Source: CAD feature listing. Evaluate the final solid. Frame: model axes, mm. A direction names the side the tool comes from. Coordinates: 2 decimals unless noted, no trailing zeros. Order: outer loops, then holes, each group sorted by start corner. A loop starts at its lowest first (then second) coordinate and runs counter-clockwise, first axis right, second up. Notation, with made-up numbers: (-14.75, 84.25) - (-7.75, 84.25) arc R8 cw to (-7.75, 99.25) - close; hole circle Ø6 at (-25.75, -10). An arc over 180 degrees is marked (long way). One line per question, with ' | ' between items. Start each with the question number.
(1) Draft query along X for faces 3 (the flat face through (-3.523, -2.068, 0.986)), 4 (the flat face through (0, -3, 0)), 5 (the cylindrical face through (-0.342, 1.442, 0.986)), 6 (the cylindrical face through (-0.09, 2.99, 0.99)). Return one class per face: +X half, -X half, draft (parallel to the pull), parting line (faces both ways), or undercut.
(2) Line query: line 1 along Z through (x, y) = (1.5, -8.75); line 2 along Y through (x, z) = (1, 0.85); line 3 along Y through (x, z) = (-1.25, 1.8). Output: solid intervals per line, ascending.
(3) Section B-B (y = -3). Return the cut outline in (x, z).
(4) Section C-C (y = 2). Return the cut outline in (x, z).
(5) Section A-A (z = 0.95). Return the cut outline in (x, y), then the cut area to 3 significant figures.
(6) Contact query for flat-ended pins moving along their axis: P1, Ø3, axis at x = 2.5, y = -1, coming from the +Z side; P2, Ø1.5, axis at x = 2.5, y = -4, coming from the +Z side. Output: stop coordinate, or through.
(7) Access query for faces 1 (the flat face through (3.5, -2.04, 0.99)), 2 (the flat face through (0, -2, 2)). Directions: +Z, -Z, +X, -X, +Y, -Y. A direction counts if a zero-diameter tool reaches every point of the face in a straight line with its end or side. Return the directions, or none.
Autodesk Inventor part; units mm, degrees
ref_plane "YZ Plane" through (0, 0, 0) normal (1, 0, 0) x (0, 1, 0)
ref_plane "XZ Plane" through (0, 0, 0) normal (0, 1, 0) x (-1, 0, 0)
ref_plane "XY Plane" through (0, 0, 0) normal (0, 0, 1) x (1, 0, 0)
sketch "Sketch1" plane through (0, 0, 0) normal (0, 0, 1) x (1, 0, 0)
  circle A0 centre (-0.0198, -0.0084) radius 1.4858
  arc A1 (0.0044, -3.1481) -> (0.0044, -8.2481) centre (0.0044, -5.6981) ccw construction
  arc A2 (0.0044, -8.2481) -> (0.0044, -3.1481) centre (0.0044, -5.6981) ccw construction
  line L0 (-5.8056, -3.1481) -> (0.0044, -3.1481) construction
  line L1 (0.0044, -8.2481) -> (-5.8056, -8.2481) construction
  line L2 (2.5544, -5.6981) -> (5.0544, -5.6981) construction
  line L3 (-5.8056, -3.1481) -> (-5.8056, -8.2481) construction
  arc A3 (2.9095, 0.6389) -> (-2.9546, 0.6139) centre (-0.0198, -0.0084) ccw
  arc A4 (-4.1081, -4.8261) -> (4.1094, -4.7911) centre (0.0044, -5.6981) ccw
  line L4 (2.9095, 0.6389) -> (4.1094, -4.7911)
  line L5 (-2.9546, 0.6139) -> (-4.1081, -4.8261)
  point P0 (0, 0)
  dimension "d0" = 2.5
  dimension "d1" = 6
extrude "Extrusion1" add sketch "Sketch1" along normal blind 2
sketch "Sketch2" plane through (0, 0, 2) normal (0, 0, 1) x (1, 0, 0)
  circle A0 centre (-0.0198, -0.0084) radius 1.4858
  arc A1 (0.0044, -3.1481) -> (0.0044, -8.2481) centre (0.0044, -5.6981) ccw construction
  arc A2 (0.0044, -8.2481) -> (0.0044, -3.1481) centre (0.0044, -5.6981) ccw construction
  line L0 (-5.8056, -3.1481) -> (0.0044, -3.1481) construction
  line L1 (0.0044, -8.2481) -> (-5.8056, -8.2481) construction
  line L2 (2.5544, -5.6981) -> (5.0544, -5.6981) construction
  line L3 (-5.8056, -3.1481) -> (-5.8056, -8.2481) construction
  arc A3 (2.9095, 0.6389) -> (-2.9546, 0.6139) centre (-0.0198, -0.0084) ccw
  arc A4 (-4.1081, -4.8261) -> (4.1094, -4.7911) centre (0.0044, -5.6981) ccw
  line L4 (2.9095, 0.6389) -> (4.1094, -4.7911)
  line L5 (-2.9546, 0.6139) -> (-4.1081, -4.8261)
  circle A5 centre (0.0044, -5.6981) radius 2.55
  point P0 (0, 0)
  point P1 (0, 0)
  dimension "d4" = 2.5
  dimension "d5" = 6
extrude "Extrusion2" add sketch "Sketch2" along normal blind 1.5 contours A5
fillet "Fillet1" radius 2.5 1 edges at (-2.5456, -5.6981, 3.5)
sketch "Sketch3" plane through (2.9095, 0.6389, 2) normal (0.9764456, 0.2157637, 0) x (0, 0, -1)
  line L0 (0, 3) -> (0, 0)
  line L1 (0, 0) -> (-1, 0)
  line L2 (-1, 0) -> (-1, -8.6875)
  line L3 (-1, -8.6875) -> (-2.9665, -8.6875)
  line L4 (-2.9665, -8.6875) -> (-2.9665, 0)
  line L5 (-2.9665, 0) -> (-1, 0)
  point P0 (2, 0.0039)
  point P1 (0, 1.2408)
  dimension "d9" = 1
extrude "Extrusion3" cut sketch "Sketch3" against normal blind 10
properties part number "Stylis holder"
Response values:
1) face 3: -X half | face 4: draft | face 5: undercut | face 6: parting line
2) line 1: z = 0 to 2 | line 2: y = -9.78 to -1.09, 1.07 to 2.81 | line 3: y = -9.71 to -0.84, 0.82 to 2.73
3) outline: (-3.72, 0) - (3.71, 0) - (3.71, 2) - (-3.72, 2) - close
4) outline: (-2.25, 0) - (2.21, 0) - (2.21, 2) - (-2.25, 2) - close
5) outline: (-4.11, -4.83) arc R4.2 ccw (long way) to (4.11, -4.79) - (2.91, 0.64) arc R3 ccw to (-2.95, 0.61) - close; hole circle Ø2.97 at (-0.02, -0.01) | area: 76.9 mm²
6) P1: stops at z = 2 | P2: stops at z = 2.49
7) face 1: +Z, -Z, +X, +Y | face 2: +Z
